Source: three-view drawing plus pictorial views. Frame: mm from the lowest corner of the part. A direction names the side the tool comes from. Coordinates: 2 decimals unless noted, no trailing zeros. Loops run counter-clockwise (first coordinate to the right, second up) from the corner with the lowest first, then second, coordinate; pieces in that order, holes last. Notation, with made-up numbers: M -17.75,-9 L 23.25,-9 A26 ccw 23.25,5 Z; hole C -37.75,0 d7. An arc over 180 degrees is marked long. Use a Markdown table: item, result. Add a question column.
1. Section A-A on z = 5.5. State how many separate pieces and enclosed holes the cut face has, then the cut area to 3 significant figures.
2. Section D-D on x = 36.5. Output: boundary loops of the cut face in (y, z).
3. Set-up query: the marked faces 1 and 2. Return all of +Z, -Z, +X, -X, +Y, -Y with unobstructed straight access to the full face (end or side cutting, diameter ignored); none if empty.
4. Section C-C on y = 11. Output: boundary loops of the cut face in (x, z).
5. Draft query along Y for the marked faces 3, 4, 5 and 6. Return one class per face: +Y half, -Y half, draft (parallel to the pull), parting line (faces both ways), or undercut.
6. Line query: L1, parallel to Y at x = 27, z = 3.75; L2, parallel to X at y = 8.5, z = 1.5; L3, parallel to Y at x = 27.5, z = 8.25 (1 decimal). Output: solid intervals per line, ascending. Write a range as [from, to].
7. Section B-B on x = 112. Output: boundary loops of the cut face in (y, z), then the cut area to 3 significant figures.
8. Pin query (flat end, axial travel): pin 1 (2.5 mm diameter, centred on x = 112, y = 6, fed in from -Z); pin 2 (12 mm diameter, centred on x = 60.5, y = 14, fed in from +Z); pin 3 (3 mm diameter, centred on y = 21.5, z = 12, fed in from -X). Return the tip coordinate at first contact, or that it passes through.
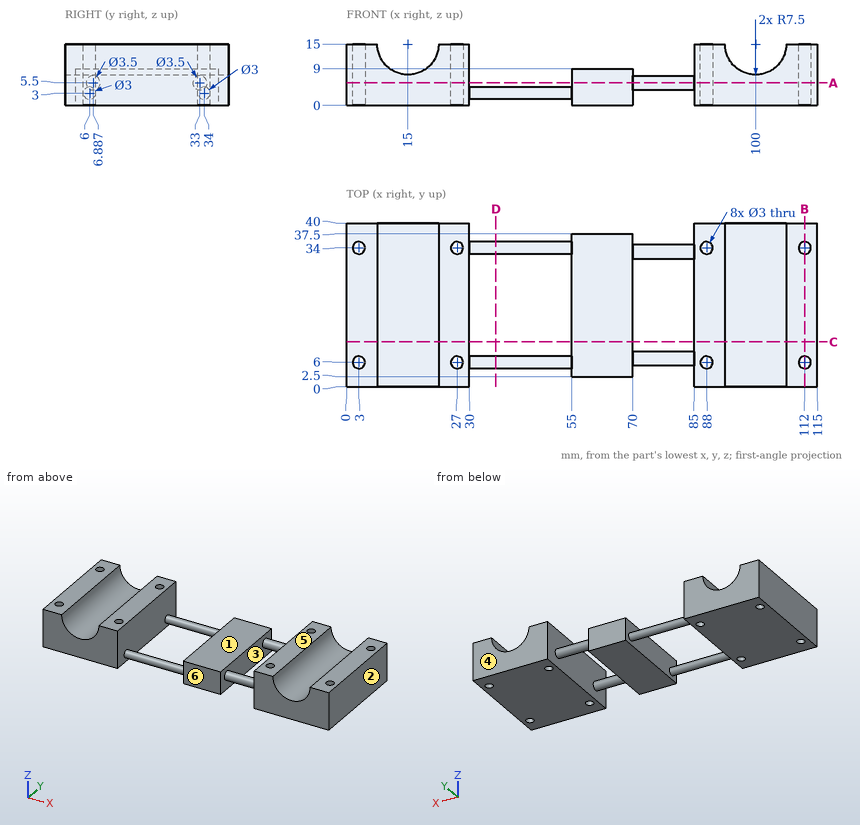
Answers below:
| question | item | result |
|---|---|---|
| 1 | separate pieces | 2 |
| 1 | enclosed holes | 9 |
| 1 | area | 2,970 mm² |
| 2 | outline | C 6,3 d3; C 34,3 d3 |
| 3 | face 1 | +Z, +Y, -Y |
| 3 | face 2 | +Z, -Z, +X, +Y, -Y |
| 4 | outline | M 0,0 L 30,0 L 30,15 L 22.5,15 A7.5 cw 7.5,15 L 0,15 Z; M 55,0 L 70,0 L 70,9 L 55,9 Z; M 85,0 L 115,0 L 115,15 L 107.5,15 A7.5 cw 92.5,15 L 85,15 Z |
| 5 | face 3 | undercut |
| 5 | face 4 | +Y half |
| 5 | face 5 | draft |
| 5 | face 6 | -Y half |
| 6 | L1 | y = [0, 4.5], [7.5, 32.5], [35.5, 40] |
| 6 | L2 | x = [0, 30], [55, 70], [85, 115] |
| 6 | L3 | y = [0, 4.6], [7.4, 32.6], [35.4, 40] |
| 7 | outline | M 0,0 L 4.5,0 L 4.5,15 L 0,15 Z; M 7.5,0 L 32.5,0 L 32.5,15 L 7.5,15 Z; M 35.5,0 L 40,0 L 40,15 L 35.5,15 Z |
| 7 | area | 510 mm² |
| 8 | pin 1 | passes through |
| 8 | pin 2 | stops at z = 9 |
| 8 | pin 3 | stops at x = 0 |
